from build123d import *

# Parameters (mm, degrees)
SKETCH1_W                = 70
SKETCH1_H                = 48
SKETCH1_W_2              = 60
SKETCH1_H_2              = 40
BOSS_EXTRUDE1_DEPTH      = 3
M3_CLEARANCE_HOLE1_D     = 3.6
M3_CLEARANCE_HOLE1_DEPTH = 9
M3_CLEARANCE_HOLE1_TIP   = 1.081549114
SKETCH6_W                = 8
SKETCH6_H                = 30
BOSS_EXTRUDE2_DEPTH      = 6
SKETCH7_W                = 54
SKETCH7_H                = 30
CUT_EXTRUDE1_DEPTH       = 43.860237983
FILLET1_R                = 2


# Read off the part's stored shape, not the designer's step: Ø1.0mm Dowel Hole1
with BuildPart() as part:
    # Sketch1 → Boss-Extrude1 (new body)
    # profile 1 of 2: a face of its own
    with BuildSketch(Plane(origin=(0, 0, 0), x_dir=(1, 0, 0), z_dir=(0, 1, 0))):
        Rectangle(SKETCH1_W, SKETCH1_H)
        Rectangle(SKETCH1_W_2, SKETCH1_H_2, mode=Mode.SUBTRACT)
    # profile 2 of 2: a face of its own
    with BuildSketch(Plane(origin=(0, 0, 0), x_dir=(1, 0, 0), z_dir=(0, 1, 0))):
        Rectangle(SKETCH1_W_2, SKETCH1_H_2)
    extrude(amount=BOSS_EXTRUDE1_DEPTH)

    # M3 Clearance Hole1
    with Locations(Plane(origin=(0, 0, 0), x_dir=(-1, 0, 0), z_dir=(0, -1, 0))):
        with Locations((30, -20), (30, 20), (-30, 20), (-30, -20)):
            Hole(M3_CLEARANCE_HOLE1_D / 2, depth=M3_CLEARANCE_HOLE1_DEPTH)
            with Locations((0, 0, -(M3_CLEARANCE_HOLE1_DEPTH + M3_CLEARANCE_HOLE1_TIP / 2))):  # 118° drill point
                Cone(0, M3_CLEARANCE_HOLE1_D / 2, M3_CLEARANCE_HOLE1_TIP, mode=Mode.SUBTRACT)

    # Sketch6 → Boss-Extrude2 (add)
    with BuildSketch(Plane.XZ):
        with Locations((-31, 0)):
            Rectangle(SKETCH6_W, SKETCH6_H)
        with Locations((31, 0)):
            Rectangle(SKETCH6_W, SKETCH6_H)
    extrude(amount=BOSS_EXTRUDE2_DEPTH)

    # Ø1.0mm Dowel Hole1 outline → Ø1.0mm Dowel Hole1 (revolve, cut)
    with BuildSketch(Plane(origin=(-32.5, 0, -12.5), x_dir=(1, 0, 0), z_dir=(0, 0, 1))):
        Polygon((1.8, 0), (0, 1.081549114), (0, -6), (1.8, -6), align=None)
    revolve(axis=Axis((-32.5, 0, -12.5), (0, 1, 0)), mode=Mode.SUBTRACT)

    # 1.0mm Dowel Hole1 2 outline → 1.0mm Dowel Hole1 2 (revolve, cut)
    with BuildSketch(Plane(origin=(32.5, 0, 12.5), x_dir=(1, 0, 0), z_dir=(0, 0, 1))):
        Polygon((1.8, 0), (0, 1.081549114), (0, -6), (1.8, -6), align=None)
    revolve(axis=Axis((32.5, 0, 12.5), (0, 1, 0)), mode=Mode.SUBTRACT)

    # 1.0mm Dowel Hole1 3 outline → 1.0mm Dowel Hole1 3 (revolve, cut)
    with BuildSketch(Plane(origin=(32.5, 0, -12.5), x_dir=(1, 0, 0), z_dir=(0, 0, 1))):
        Polygon((1.8, 0), (0, 1.081549114), (0, -6), (1.8, -6), align=None)
    revolve(axis=Axis((32.5, 0, -12.5), (0, 1, 0)), mode=Mode.SUBTRACT)

    # 1.0mm Dowel Hole1 4 outline → 1.0mm Dowel Hole1 4 (revolve, cut)
    with BuildSketch(Plane(origin=(-32.5, 0, 12.5), x_dir=(1, 0, 0), z_dir=(0, 0, 1))):
        Polygon((1.8, 0), (0, 1.081549114), (0, -6), (1.8, -6), align=None)
    revolve(axis=Axis((-32.5, 0, 12.5), (0, 1, 0)), mode=Mode.SUBTRACT)

    # 1.0mm Dowel Hole1 5 outline → 1.0mm Dowel Hole1 5 (revolve, cut)
    with BuildSketch(Plane.XY):
        Polygon((1.8, 0), (0, 1.081549114), (0, 0), align=None)
    revolve(axis=Axis((0, 0, 0), (0, 1, 0)), mode=Mode.SUBTRACT)

    # Sketch7 → Cut-Extrude1 (cut, through all)
    with BuildSketch(Plane.XZ):
        Rectangle(SKETCH7_W, SKETCH7_H)
    extrude(amount=-CUT_EXTRUDE1_DEPTH, mode=Mode.SUBTRACT)

    # Fillet1
    fillet1_edges = [part.edges().sort_by_distance(p)[0] for p in [
        (-27, 1.5, -15),
        (-27, 1.5, 15),
        (27, 1.5, 15),
        (27, 1.5, -15),
        (-35, 1.5, -24),
        (35, 1.5, -24),
        (35, 1.5, 24),
        (-35, 1.5, 24),
    ]]
    fillet(fillet1_edges, radius=FILLET1_R)


solid = part.part
Part model, mm, in its own coordinate system. A direction names the side the tool comes from. Give positions to 0.01 mm unless a question says otherwise; leave off trailing zeros. Order: outer loops, then holes, each group sorted by start corner. A loop starts at its lowest first (then second) coordinate and runs counter-clockwise, first axis right, second up. Notation, with made-up numbers: (-13, 85.5) - (10, 85.5) arc R34 ccw to (10, 123.5) - close; hole circle Ø9 at (73.25, -37.5). An arc over 180 degrees is marked (long way). Use a Markdown table: item, result.
1) Saw through at B-B on z = 20. List the corners of the cut face in (x, y), plus the area to 3 significant figures.
Checked values:
| item | result |
|---|---|
| outline | (-35, 0) - (-31.8, 0) - (-31.8, 3) - (-35, 3) - close; (-28.2, 0) - (28.2, 0) - (28.2, 3) - (-28.2, 3) - close; (31.8, 0) - (35, 0) - (35, 3) - (31.8, 3) - close |
| area | 188 mm² |
2) Two-plate mould, pull along Z, no slides. Class faces 1 (the flat face through (0, 3, -16)), 2 (the flat face through (27, -2, 0)), 3 (the cylindrical face through (34.43, 1.52, -23.4)): +Z half, -Z half, draft (parallel to the pull), parting line (faces both ways), or undercut.
Checked values:
| item | result |
|---|---|
| face 1 | draft |
| face 2 | undercut |
| face 3 | -Z half |
3) Probe L1, parallel to X at y = -2.25, z = -12.5; L2, parallel to X at y = 2.05, z = 20; L3, parallel to Z at x = 30, y = 0.7. List the from-to ranges inside material, lowest first. Write a range as from..to.
Checked values:
| item | result |
|---|---|
| L1 | -35..-34.3, -30.7..-27, 27..30.7, 34.3..35 |
| L2 | -35..-31.8, -28.2..28.2, 31.8..35 |
| L3 | -24..-21.8, -18.2..18.2, 21.8..24 |
4) Flat gauge pins, fed straight in: P1, Ø3, axis at x = -30, z = -20, coming from the -Y side; P2, Ø4, axis at x = 1, z = -15, coming from the -Y side; P3, Ø3, axis at x = -33, y = -2.5, coming from the -Z side; P4, Ø3, axis at x = 33, y = -2, coming from the +Z side. Where does each tip first touch, or does it go through?
Checked values:
| item | result |
|---|---|
| P1 | through |
| P2 | y = 0 |
| P3 | z = -15 |
| P4 | z = 15 |
5) Saw through at D-D on x = 30. List the corners of the cut face in (y, z).
Checked values:
| item | result |
|---|---|
| outline | (-6, -15) - (0, -15) - (0, -18.2) - (3, -18.2) - (3, 18.2) - (0, 18.2) - (0, 15) - (-6, 15) - close; (0, -24) - (3, -24) - (3, -21.8) - (0, -21.8) - close; (0, 21.8) - (3, 21.8) - (3, 24) - (0, 24) - close |
6) 3-axis set-ups, long thin cutter, end or side, ignore diameter. For faces 4 (the cylindrical face through (-30.783, -2.958, -13.041)), 5 (the cylindrical face through (26.4, 1.52, 14.43)), 6 (the flat face through (-31, -3, -15)): which of +Z, -Z, +X, -X, +Y, -Y reach the whole face in a straight line?
Checked values:
| item | result |
|---|---|
| face 4 | -Y |
| face 5 | +Y, -Y |
| face 6 | -Z, +X, -X, -Y |
7) Saw through at C-C on x = -4.5. List the corners of the cut face in (y, z).
Checked values:
| item | result |
|---|---|
| outline | (0, -24) - (3, -24) - (3, -15) - (0, -15) - close; (0, 15) - (3, 15) - (3, 24) - (0, 24) - close |
8) Saw through at A-A on y = -0.75. List the corners of the cut face in (x, z), plus the area to 3 significant figures.
Checked values:
| item | result |
|---|---|
| outline | (-35, -15) - (-27, -15) - (-27, 15) - (-35, 15) - close; (27, -15) - (35, -15) - (35, 15) - (27, 15) - close; hole circle Ø3.6 at (-32.5, -12.5); hole circle Ø3.6 at (-32.5, 12.5); hole circle Ø3.6 at (32.5, -12.5); hole circle Ø3.6 at (32.5, 12.5) |
| area | 439 mm² |
